Can you work these out from the model? Positions are in its coordinate system, mm. Face numbers are marked on the shaded views. Round coordinates to 2 decimals unless told otherwise and drop trailing zeros. Loops run counter-clockwise (first coordinate to the right, second up) from the corner with the lowest first, then second, coordinate; pieces in that order, holes last. Notation, with made-up numbers: (-12, 29.5) -> (28, 29.5) arc R22 cw to (28, 55.5) -> close; hole circle Ø3 at (71.5, -32). An arc over 180 degrees is marked (long way). Use a Markdown table: item, result.
from build123d import *

# Parameters (mm, degrees)
SKETCH1_R           = 27.5
SKETCH1_R_2         = 26
BOSS_EXTRUDE1_DEPTH = 20
SKETCH1_3_R         = 26
BOSS_EXTRUDE2_DEPTH = 3
BOSS_EXTRUDE3_START = -7
SKETCH1_4_R         = 27.5
SKETCH1_4_W         = 0.030258968
SKETCH1_4_H         = 20
BOSS_EXTRUDE3_DEPTH = 7
SKETCH4_W           = 11
SKETCH4_H           = 3.5
CUT_EXTRUDE3_DEPTH  = 2.5
SKETCH4_2_W         = 11
SKETCH4_2_H         = 3.5
CUT_EXTRUDE4_DEPTH  = 51.621141828


with BuildPart() as part:
    # Sketch1 → Boss-Extrude1 (new body)
    with BuildSketch(Plane(origin=(0, 0, 0), x_dir=(1, 0, 0), z_dir=(0, 1, 0))):
        with Locations(Location((0, 0, 0), (0, 0, 270))):
            Circle(SKETCH1_R)
        with Locations(Location((0, 0, 0), (0, 0, 270))):
            Circle(SKETCH1_R_2, mode=Mode.SUBTRACT)
    extrude(amount=BOSS_EXTRUDE1_DEPTH)

    # Sketch1_3 → Boss-Extrude2 (add)
    with BuildSketch(Plane(origin=(0, 0, 0), x_dir=(1, 0, 0), z_dir=(0, 1, 0))):
        with Locations(Location((0, 0, 0), (0, 0, 270))):
            Circle(SKETCH1_3_R)
        Polygon((22.469741032, -10), (-22.5, -10), (-22.530258968, -10), (-22.530258968, 10), (-22.5, 10), (22.469741032, 10), align=None, mode=Mode.SUBTRACT)
    extrude(amount=BOSS_EXTRUDE2_DEPTH)

    # Sketch1_4 → Boss-Extrude3 (add)
    with BuildSketch(Plane(origin=(0, 0, 0), x_dir=(1, 0, 0), z_dir=(0, 1, 0)).offset(BOSS_EXTRUDE3_START)):
        Circle(SKETCH1_4_R)
        with Locations((-22.515129484, 0)):
            Rectangle(SKETCH1_4_W, SKETCH1_4_H, mode=Mode.SUBTRACT)
    extrude(amount=BOSS_EXTRUDE3_DEPTH)

    # Sketch4 → Cut-Extrude3 (cut, symmetric)
    with BuildSketch(Plane(origin=(0, 0, 10), x_dir=(-1, 0, 0), z_dir=(0, 0, -1))):
        with Locations((0, -1.75)):
            Rectangle(SKETCH4_W, SKETCH4_H)
    extrude(amount=CUT_EXTRUDE3_DEPTH, both=True, mode=Mode.SUBTRACT)

    # Sketch4_2 → Cut-Extrude4 (cut, through all)
    with BuildSketch(Plane(origin=(0, 0, 10), x_dir=(-1, 0, 0), z_dir=(0, 0, -1))):
        with Locations((0, -1.75)):
            Rectangle(SKETCH4_2_W, SKETCH4_2_H)
    extrude(amount=-CUT_EXTRUDE4_DEPTH, mode=Mode.SUBTRACT)


solid = part.part
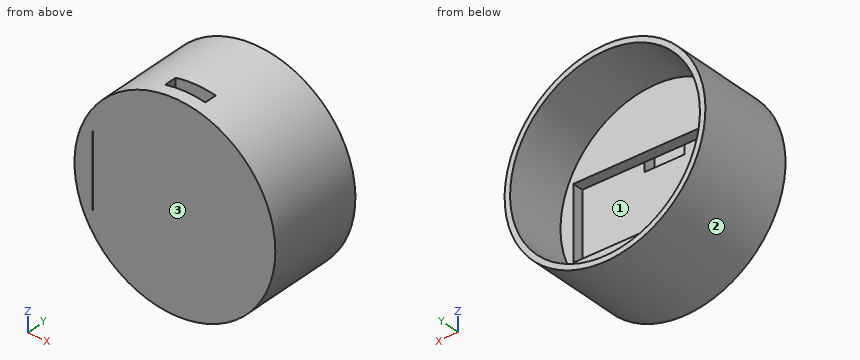
1. I want a section at A-A (z = -7.5). Please give me the cut outline in (x, y), plus the area to 3 significant figures.
Answer sheet:
| item | result |
|---|---|
| outline | (-26.46, -7) -> (-22.53, -7) -> (-22.53, 3) -> (-24.89, 3) -> (-24.89, 20) -> (-26.46, 20) -> close; (-22.5, -7) -> (26.46, -7) -> (26.46, 20) -> (24.89, 20) -> (24.89, 3) -> (22.47, 3) -> (22.47, 0) -> (-22.5, 0) -> close |
| area | 447 mm² |
2. If we mould it in two halves opening along Z, with no side actions, what happens to the marked faces 1, 2 and 3? For each: +Z half, -Z half, draft (parallel to the pull), parting line (faces both ways), or undercut.
Answer sheet:
| item | result |
|---|---|
| face 1 | undercut |
| face 2 | parting line |
| face 3 | draft |
3. I want a section at B-B (y = 6). Please give me the cut outline in (x, z), plus the area to 3 significant figures.
Answer sheet:
| item | result |
|---|---|
| outline | circle Ø55 at (0, 0); hole circle Ø52 at (0, 0) |
| area | 252 mm² |
4. I want a section at C-C (z = -1.5). Please give me the cut outline in (x, y), plus the area to 3 significant figures.
Answer sheet:
| item | result |
|---|---|
| outline | (-27.46, -7) -> (-22.53, -7) -> (-22.53, 3) -> (-25.96, 3) -> (-25.96, 20) -> (-27.46, 20) -> close; (-22.5, -7) -> (27.46, -7) -> (27.46, 20) -> (25.96, 20) -> (25.96, 3) -> (22.47, 3) -> (22.47, 0) -> (-22.5, 0) -> close |
| area | 465 mm² |
5. I need wall thicknesses on line 1 (X direction, y = 15, z = 0); line 2 (Y direction, x = 3, z = 14.5); line 3 (Y direction, x = -20, z = 2). Which ranges of each line are inside material? Lowest first, please.
Answer sheet:
| item | result |
|---|---|
| line 1 | x = -27.5 to -26, 26 to 27.5 |
| line 2 | y = -7 to -3.5, 0 to 3 |
| line 3 | y = -7 to 0 |
6. I want a section at D-D (x = -16). Please give me the cut outline in (y, z).
Answer sheet:
| item | result |
|---|---|
| outline | (-7, -22.37) -> (20, -22.37) -> (20, -20.49) -> (3, -20.49) -> (3, -10) -> (0, -10) -> (0, 10) -> (3, 10) -> (3, 20.49) -> (20, 20.49) -> (20, 22.37) -> (-7, 22.37) -> close |
7. Will these pins go through, and if not, where does the flat tip stop? pin 1 Ø5 at (x, y) = (1, -3.5) entering from -Z; pin 2 Ø1.5 at (x, y) = (-5, 13.5) entering from -Z; pin 3 Ø3 at (x, y) = (0.5, -1) entering from +Z; pin 4 Ø6 at (x, y) = (15.5, 17.5) entering from +Z.
Answer sheet:
| item | result |
|---|---|
| pin 1 | stops at z = -27.5 |
| pin 2 | stops at z = -27.17 |
| pin 3 | stops at z = 27.5 |
| pin 4 | stops at z = 24.49 |
